Part print with two shaded views. Sizes in mm from the minimum x, y, z corner. A direction names the side the tool comes from. Coordinates: 2 decimals unless noted, no trailing zeros. Write each loop counter-clockwise with the first axis right and the second up, starting at its lowest first coordinate (ties: lowest second). Pieces come first, ordered by that corner, then holes. Notation, with made-up numbers: (72, -8.5) - (128, -8.5) arc R34 cw to (128, 22.5) - close; hole circle Ø10 at (11.5, 36.25). An arc over 180 degrees is marked (long way). Answer in a Markdown table with one row per item. Add a question column.
Q1. 3-axis set-ups, long thin cutter, end or side, ignore diameter. For the marked faces 5, 6, 7, 8 and 9: which of +Z, -Z, +X, -X, +Y, -Y reach the whole face in a straight line?
Q2. Drill centre lines: line 1 along Z through (x, y) = (15, 3.15); line 2 along X through (y, z) = (39, 108.5); line 3 along X through (y, z) = (50.65, 28.5). Where is each one in solid material? Low to high. Write a range as from..to.
Q3. Band-saw the part on D-D (y = 33). List the corners of the cut face in (x, z), and give its area (3 significant figures).
Q4. Band-saw the part on A-A (x = 121). List the corners of the cut face in (y, z).
Q5. Band-saw the part on B-B (z = 80). List the corners of the cut face in (x, y).
Q6. Band-saw the part on C-C (x = 59). List the corners of the cut face in (y, z), and give its area (3 significant figures).
Q7. Pin check, flat tips, straight feed: pin 1 (4 mm diameter, centred on x = 30, y = 4, fed in from +Z); pin 2 (1 mm diameter, centred on y = 36.5, z = 117, fed in from -X). Stop position of each tip, or through.
Q8. Two-plate mould, pull along Y, no slides. Class the marked faces 1, 2, 3 and 4: +Y half, -Y half, draft (parallel to the pull), parting line (faces both ways), or undercut.
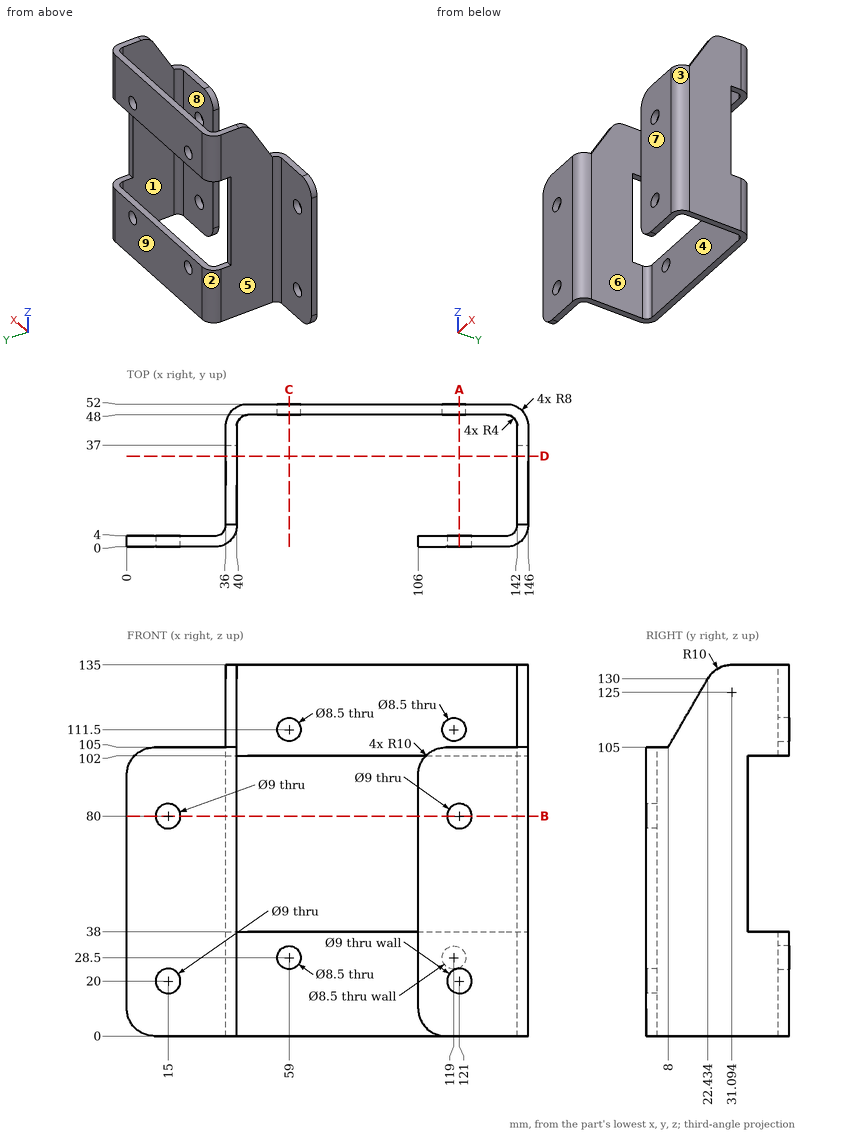
Checked values:
| question | item | result |
|---|---|---|
| 1 | face 5 | +Z, -Z, -X, +Y |
| 1 | face 6 | +Z, -Z, -Y |
| 1 | face 7 | +Z, -Z, +X, -X, -Y |
| 1 | face 8 | +Z, -Z |
| 1 | face 9 | +Z, -Z, +X, -X, +Y |
| 2 | line 1 | z = 0..15.5, 24.5..75.5, 84.5..105 |
| 2 | line 2 | x = 36..40, 142..146 |
| 2 | line 3 | x = 39.55..54.75, 63.25..114.75, 123.25..142.45 |
| 3 | outline | (36, 0) - (40, 0) - (40, 135) - (36, 135) - close; (142, 0) - (146, 0) - (146, 135) - (142, 135) - close |
| 3 | area | 1,080 mm² |
| 4 | outline | (0, 0) - (4, 0) - (4, 15.5) - (0, 15.5) - close; (0, 24.5) - (4, 24.5) - (4, 75.5) - (0, 75.5) - close; (0, 84.5) - (4, 84.5) - (4, 105) - (0, 105) - close; (48, 0) - (52, 0) - (52, 24.75) - (48, 24.75) - close; (48, 32.25) - (52, 32.25) - (52, 38) - (48, 38) - close; (48, 102) - (52, 102) - (52, 107.75) - (48, 107.75) - close; (48, 115.25) - (52, 115.25) - (52, 135) - (48, 135) - close |
| 5 | outline | (0, 0) - (10.5, 0) - (10.5, 4) - (0, 4) - close; (19.5, 0) - (32, 0) arc R8 ccw to (40, 8) - (40, 37) - (36, 37) - (36, 8) arc R4 cw to (32, 4) - (19.5, 4) - close; (106, 0) - (116.5, 0) - (116.5, 4) - (106, 4) - close; (125.5, 0) - (138, 0) arc R8 ccw to (146, 8) - (146, 37) - (142, 37) - (142, 8) arc R4 cw to (138, 4) - (125.5, 4) - close |
| 6 | outline | (48, 0) - (52, 0) - (52, 24.25) - (48, 24.25) - close; (48, 32.75) - (52, 32.75) - (52, 38) - (48, 38) - close; (48, 102) - (52, 102) - (52, 107.25) - (48, 107.25) - close; (48, 115.75) - (52, 115.75) - (52, 135) - (48, 135) - close |
| 6 | area | 216 mm² |
| 7 | pin 1 | stops at z = 105 |
| 7 | pin 2 | stops at x = 36 |
| 8 | face 1 | undercut |
| 8 | face 2 | +Y half |
| 8 | face 3 | -Y half |
| 8 | face 4 | undercut |
